from build123d import *

# Parameters (mm, degrees)
F0_W     = 317.5
F0_H     = 317.5
F0_W_2   = 304.8
F0_H_2   = 304.8
F1_DEPTH = 38.1
F2_R     = 25.4
F3_D     = 12.7
F4_D     = 12.7


with BuildPart() as f1:
    # F0 (on Front) → F1 (new body)
    with BuildSketch(Plane.XZ):
        Rectangle(F0_W, F0_H)
        Rectangle(F0_W_2, F0_H_2, mode=Mode.SUBTRACT)
    extrude(amount=F1_DEPTH)

    # F2
    f2_edges = [f1.edges().sort_by_distance(p)[0] for p in [
        (152.4, -19.05, -152.4),
        (-152.4, -19.05, -152.4),
        (-152.4, -19.05, 152.4),
        (152.4, -19.05, 152.4),
        (158.75, -19.05, -158.75),
        (158.75, -19.05, 158.75),
        (-158.75, -19.05, 158.75),
        (-158.75, -19.05, -158.75),
    ]]
    fillet(f2_edges, radius=F2_R)

    # F3 (through all)
    with Locations(Plane.YZ):
        with Locations((-19.05, 0)):
            Hole(F3_D / 2)

    # F4 (through all)
    with Locations(Plane(origin=(0, 0, 0), x_dir=(0, 1, 0), z_dir=(-1, 0, 0))):
        with Locations((-19.05, 0)):
            Hole(F4_D / 2)


solid = f1.part
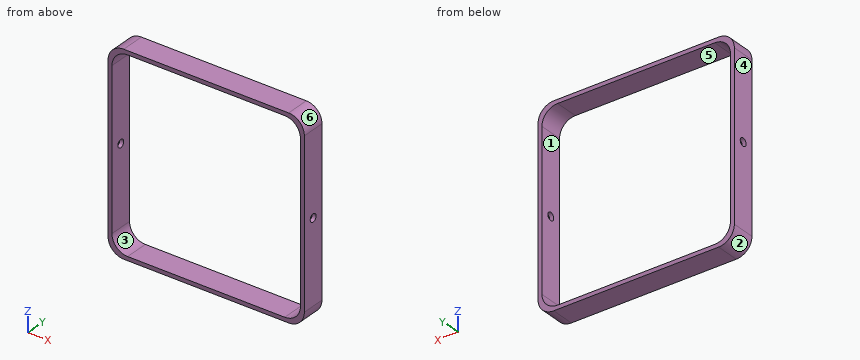
Here's how the part is built. I have some questions about the finished solid (model axes, mm). Face numbers are marked on the shaded views. A direction names the side the tool comes from. Round coordinates to 2 decimals unless told otherwise and drop trailing zeros. Order: outer loops, then holes, each group sorted by start corner. A loop starts at its lowest first (then second) coordinate and runs counter-clockwise, first axis right, second up. Notation, with made-up numbers: (51.25, -16) -> (94.25, -16) arc R21 cw to (94.25, -1) -> close; hole circle Ø11 at (8.25, -17.75). An arc over 180 degrees is marked (long way). Return JSON: item names as keys, results as strings.
Q1. Which directions (+Z, -Z, +X, -X, +Y, -Y) give clear straight access to the entire face, cutting with the end or side of a thin tool? Please do the marked faces 5 and 6.
Filled sheet:
{"face 5": "+Y, -Y", "face 6": "+Z, +X, +Y, -Y"}
Q2. If we section it at C-C on x = -47: List the corners of the cut face in (y, z) for me.
Filled sheet:
{"outline": "(-38.1, -158.75) -> (0, -158.75) -> (0, -152.4) -> (-38.1, -152.4) -> close; (-38.1, 152.4) -> (0, 152.4) -> (0, 158.75) -> (-38.1, 158.75) -> close"}
Q3. I need wall thicknesses on line 1 along X through (y, z) = (-23.5, -113.5); line 2 along Z through (x, y) = (-154.25, -19.05). Which ranges of each line are inside material? Lowest first, please. Write a range as from..to.
Filled sheet:
{"line 1": "x = -158.75..-152.4, 152.4..158.75", "line 2": "z = -147.78..-6.35, 6.35..147.78"}
Q4. For pin 1 Ø14.5 at (y, z) = (-19.05, 0) entering from -X, with a flat end and sliding along its axis, tell me the tip position at first contact or that it passes through.
Filled sheet:
{"pin 1": "stops at x = -158.75"}
Q5. If we section it at A-A on z = 0: List the corners of the cut face in (x, y) for me.
Filled sheet:
{"outline": "(-158.75, -38.1) -> (-152.4, -38.1) -> (-152.4, -25.4) -> (-158.75, -25.4) -> close; (-158.75, -12.7) -> (-152.4, -12.7) -> (-152.4, 0) -> (-158.75, 0) -> close; (152.4, -38.1) -> (158.75, -38.1) -> (158.75, -25.4) -> (152.4, -25.4) -> close; (152.4, -12.7) -> (158.75, -12.7) -> (158.75, 0) -> (152.4, 0) -> close"}
Q6. If we mould it in two halves opening along Z, with no side actions, what happens to the marked faces 1, 2, 3 and 4? For each: released by +Z, released by -Z, zero draft, split by the parting line, or undercut.
Filled sheet:
{"face 1": "undercut", "face 2": "released by -Z", "face 3": "undercut", "face 4": "zero draft"}
Q7. If we section it at D-D on z = -68: List the corners of the cut face in (x, y) for me.
Filled sheet:
{"outline": "(-158.75, -38.1) -> (-152.4, -38.1) -> (-152.4, 0) -> (-158.75, 0) -> close; (152.4, -38.1) -> (158.75, -38.1) -> (158.75, 0) -> (152.4, 0) -> close"}
Q8. If we section it at B-B on y = -19.05: List the corners of the cut face in (x, z) for me.
Filled sheet:
{"outline": "(-158.75, -133.35) arc R25.4 ccw to (-133.35, -158.75) -> (133.35, -158.75) arc R25.4 ccw to (158.75, -133.35) -> (158.75, -6.35) -> (152.4, -6.35) -> (152.4, -127) arc R25.4 cw to (127, -152.4) -> (-127, -152.4) arc R25.4 cw to (-152.4, -127) -> (-152.4, -6.35) -> (-158.75, -6.35) -> close; (-158.75, 6.35) -> (-152.4, 6.35) -> (-152.4, 127) arc R25.4 cw to (-127, 152.4) -> (127, 152.4) arc R25.4 cw to (152.4, 127) -> (152.4, 6.35) -> (158.75, 6.35) -> (158.75, 133.35) arc R25.4 ccw to (133.35, 158.75) -> (-133.35, 158.75) arc R25.4 ccw to (-158.75, 133.35) -> close"}
